from build123d import *

# Parameters (mm, degrees)
F1_DEPTH  = 75
F3_DEPTH  = 210
F3_TAPER  = 1.5
F7_DEPTH  = 75
F10_W     = 10
F10_H     = 3
F11_DEPTH = 65


# Not quite as in the source:
# - a feature names something its author has since deleted; it is built from what else it names


with BuildPart() as f1:
    # F0 (on Front) → F1 (new body)
    with BuildSketch(Plane.XZ):
        Polygon((-10, -17.3205080757), (10, -17.3205080757), (20, 0), (10, 17.3205080757), (-10, 17.3205080757), (-20, 0), align=None)
    extrude(amount=-F1_DEPTH)

    # F2 (on face) → F3 (join)
    with BuildSketch(Plane.XZ):
        Polygon((10, -17.3205080757), (20, 0), (-20, 0), (-10, -17.3205080757), align=None)
    extrude(amount=F3_DEPTH, taper=F3_TAPER)

    # F4 (on face) → F6 section 0
    with BuildSketch(Plane.XZ.offset(210)):
        Polygon((-10.4753772138, -5.4990435295), (10.4753772138, -5.4990435295), (6.8251257379, 0.8233774871), (-6.8251257379, 0.8233774871), align=None)
    # F5 (on face) → F6 section 1
    with BuildSketch(Plane.XZ):
        Polygon((-10, 17.3205080757), (-20, 0), (20, 0), (10, 17.3205080757), align=None)
    loft()

    # F0 (on Front) → F7 (join, through all)
    with BuildSketch(Plane.XZ):
        Polygon((-10, 17.3205080757), (10, 17.3205080757), (8.5, 23.3205080757), (-8.5, 23.3205080757), align=None)
    extrude(amount=-F7_DEPTH)

    # F10 (on offset) → F11 (cut)
    with BuildSketch(Plane.XZ.offset(-5)):
        with Locations((0, 21.8205080757)):
            Rectangle(F10_W, F10_H)
    extrude(amount=-F11_DEPTH, mode=Mode.SUBTRACT)

    # F14: sweep along a path in F13
    with BuildLine(Plane.YZ) as f14_path:
        Line((-7.1518244222, 23.3403816819), (-35.0594446063, 13.796761632))
    # F12 (on offset) → F14 (sweep)
    with BuildSketch(Plane.XZ.offset(7)):
        Polygon((-8.5, 23.3205080757), (-15.4033075124, 4.9551053697), (16.0198838661, 4.9551053697), (8.5, 23.3205080757), align=None)
    sweep(path=f14_path.line)

    # F16: sweep along a path in F15
    with BuildLine(Plane.YZ) as f16_path:
        Line((-6.9480864331, 23.3692936599), (0, 23.3692936599))
    # F12 (on offset) → F16 (sweep)
    with BuildSketch(Plane.XZ.offset(7)):
        Polygon((-8.5, 23.3205080757), (-15.4033075124, 4.9551053697), (16.0198838661, 4.9551053697), (8.5, 23.3205080757), align=None)
    sweep(path=f16_path.line)


solid = f1.part
Check sheet for the modelled part. Datum: model origin and axes. Units: mm. A direction names the side the tool comes from. Round coordinates to 2 decimals unless told otherwise and drop trailing zeros. Order: outer loops, then holes, each group sorted by start corner. A loop starts at its lowest first (then second) coordinate and runs counter-clockwise, first axis right, second up.
(1) Scan lines: probe 1 along X at (y, z) = (39, 7); probe 2 along X at (y, z) = (50.5, 13); probe 3 along Z at (x, y) = (5, -135). Record each from-to range of solid material in increasing order.
(2) Cross-section at A-A, the plane y = 45. Enter the section's corners in (x, z), and give its area (3 significant figures).
(3) Access from +Z, -Z, +X, -X, +Y, -Y to the whole of each face (thin tool, end or side, straight path). Record for faces 1 (the flat face through (0, 37, -17.321)), 2 (the flat face through (-9.24, 36.98, 20.36)), 3 (the flat face through (15.07, 36.98, 8.54)), 4 (the flat face through (0, 37, 20.321)), 5 (the flat face through (6, 37, 23.321)).
(4) Go/stop test with flat-tipped pins: P1, Ø4, axis at x = 6.5, y = -81.5, coming from the -Z side; P2, Ø1.5, axis at x = 6, y = -112.5, coming from the +Z side; P3, Ø1, axis at x = 11.5, y = -18.5, coming from the +Z side. Record where each tip stops, or that it passes through.
Check sheet entries:
1. probe 1: x = -15.96 to 15.96
1. probe 2: x = -12.49 to 12.49
1. probe 3: z = -13.79 to 6.72
2. outline: (-20, 0) - (-10, -17.32) - (10, -17.32) - (20, 0) - (10, 17.32) - (8.5, 23.32) - (5, 23.32) - (5, 20.32) - (-5, 20.32) - (-5, 23.32) - (-8.5, 23.32) - (-10, 17.32) - close
2. area: 1,120 mm2
3. face 1: -Z, +X, -X, +Y, -Y
3. face 2: +Z, -X, +Y
3. face 3: +Z, +X, +Y
3. face 4: +Z
3. face 5: +Z, +X, -X, +Y, -Y
4. P1: stops at z = -15.24
4. P2: stops at z = 8.54
4. P3: stops at z = 13.65
